```python
from build123d import *

# Parameters (mm, degrees)
BOSS_EXTRUDE1_DEPTH = 35.687
FILLET1_R           = 6.35
SKETCH3_R           = 4.1656
CUT_EXTRUDE1_DEPTH  = 114.518465322
CUT_EXTRUDE2_REACH  = 115.518
SKETCH4_R           = 4.1656


with BuildPart() as part:
    # Sketch2 → Boss-Extrude1 (new, symmetric)
    with BuildSketch(Plane.XY):
        with BuildLine():
            Line((0, 0), (0, 76.2))
            Line((0, 76.2), (6.35, 76.2))
            Line((6.35, 76.2), (6.35, 14.2748))
            ThreePointArc((6.35, 14.2748), (8.67112018, 8.67112018), (14.2748, 6.35))
            Line((14.2748, 6.35), (76.2, 6.35))
            Line((76.2, 6.35), (76.2, 0))
            Line((76.2, 0), (0, 0))
        make_face()
    extrude(amount=BOSS_EXTRUDE1_DEPTH, both=True)

    # Fillet1
    fillet1_edges = [part.edges().sort_by_distance(p)[0] for p in [
        (76.2, 6.35, 0),
        (6.35, 76.2, 0),
    ]]
    fillet(fillet1_edges, radius=FILLET1_R - 0.0001)  # a hair under: the kernel refuses the full size

    # Sketch3 → Cut-Extrude1 (cut, through all)
    with BuildSketch(Plane.ZY):
        with Locations(Location((-19.05, 57.15, 0), (0, 0, 270))):
            Circle(SKETCH3_R)
        with Locations(Location((-19.05, 19.05, 0), (0, 0, 270))):
            Circle(SKETCH3_R)
        with Locations(Location((19.05, 19.05, 0), (0, 0, 270))):
            Circle(SKETCH3_R)
        with Locations(Location((19.05, 57.15, 0), (0, 0, 270))):
            Circle(SKETCH3_R)
    extrude(amount=-CUT_EXTRUDE1_DEPTH, mode=Mode.SUBTRACT)

    # Sketch4 → Cut-Extrude2 (cut, up to next)
    with BuildSketch(Plane.XZ, mode=Mode.PRIVATE) as cut_extrude2_sk1:
        with Locations((57.15, 19.05)):
            Circle(SKETCH4_R)
    cut_extrude2_tool1 = extrude(cut_extrude2_sk1.sketch, amount=-CUT_EXTRUDE2_REACH, mode=Mode.PRIVATE) & part.part
    # Sketch4 → Cut-Extrude2 (cut, up to next)
    with BuildSketch(Plane.XZ, mode=Mode.PRIVATE) as cut_extrude2_sk2:
        with Locations(Location((19.05, -19.05, 0), (0, 0, 270))):
            Circle(SKETCH4_R)
    cut_extrude2_tool2 = extrude(cut_extrude2_sk2.sketch, amount=-CUT_EXTRUDE2_REACH, mode=Mode.PRIVATE) & part.part
    # Sketch4 → Cut-Extrude2 (cut, up to next)
    with BuildSketch(Plane.XZ, mode=Mode.PRIVATE) as cut_extrude2_sk3:
        with Locations(Location((57.15, -19.05, 0), (0, 0, 270))):
            Circle(SKETCH4_R)
    cut_extrude2_tool3 = extrude(cut_extrude2_sk3.sketch, amount=-CUT_EXTRUDE2_REACH, mode=Mode.PRIVATE) & part.part
    # Sketch4 → Cut-Extrude2 (cut, up to next)
    with BuildSketch(Plane.XZ, mode=Mode.PRIVATE) as cut_extrude2_sk4:
        with Locations((19.05, 19.05)):
            Circle(SKETCH4_R)
    cut_extrude2_tool4 = extrude(cut_extrude2_sk4.sketch, amount=-CUT_EXTRUDE2_REACH, mode=Mode.PRIVATE) & part.part
    add(cut_extrude2_tool1.solids().sort_by_distance((57.15, 0, 19.05))[0], mode=Mode.SUBTRACT)
    add(cut_extrude2_tool2.solids().sort_by_distance((19.05, 0, -19.05))[0], mode=Mode.SUBTRACT)
    add(cut_extrude2_tool3.solids().sort_by_distance((57.15, 0, -19.05))[0], mode=Mode.SUBTRACT)
    add(cut_extrude2_tool4.solids().sort_by_distance((19.05, 0, 19.05))[0], mode=Mode.SUBTRACT)


solid = part.part
```
Geometry: final body of the model. Coordinates: model frame, mm. A direction names the side the tool comes from. Coordinates: 2 decimals unless noted, no trailing zeros. Order: outer loops, then holes, each group sorted by start corner. A loop starts at its lowest first (then second) coordinate and runs counter-clockwise, first axis right, second up. Notation, with made-up numbers: M 2.25,64.25 L 61.25,64.25 A30 ccw 61.25,102.25 Z; hole C 37.25,26 d4. An arc over 180 degrees is marked long. Answer in a Markdown table with one row per item. Add a question column.
Q1. Contact query for flat-ended pins moving along their axis: P1, Ø9.5, axis at y = 19.05, z = 19.05, coming from the +X side; P2, Ø5, axis at x = 19.05, z = 19.05, coming from the +Y side; P3, Ø8, axis at x = 38.5, z = -9, coming from the -Y side. Output: stop coordinate, or through.
Q2. Line query: L1, parallel to Z at x = 57, y = 3; L2, parallel to Y at x = 2, z = -19; L3, parallel to Y at x = 32, z = 16. Output: solid intervals per line, ascending.
Q3. Mould query, pull axis X, two halves, no side actions, for faces 3 (the cylindrical face through (60.66, 3.13, -21.29)), 4 (the cylindrical face through (74.39, 4.44, 0.5)), 5 (the cylindrical face through (3.131, 58.053, 14.983)). Classes: released by +X, released by -X, zero draft, split by the parting line, or undercut.
Q4. Section query A-A on x = 57.15. Return the cut outline in (y, z), and give its area (3 significant figures).
Q5. Section query B-B on z = -19.05. Count the separate pieces of the cut face and the enclosed holes in it, and give its area (3 significant figures).
Q6. Reachability of faces 1 (the flat face through (6.35, 42, 0)), 2 (the cylindrical face through (53.84, 3.13, 16.52)) from +Z, -Z, +X, -X, +Y, -Y: full face, straight path, thin tool, end or side. Return the list, or none.
Completed:
| question | item | result |
|---|---|---|
| 1 | P1 | stops at x = 6.35 |
| 1 | P2 | passes through |
| 1 | P3 | stops at y = 0 |
| 2 | L1 | z = -35.69 to -23.21, -14.89 to 14.89, 23.21 to 35.69 |
| 2 | L2 | y = 0 to 14.88, 23.22 to 52.98, 61.32 to 75.88 |
| 2 | L3 | y = 0 to 6.35 |
| 3 | face 3 | undercut |
| 3 | face 4 | released by +X |
| 3 | face 5 | zero draft |
| 4 | outline | M 0,-35.69 L 6.35,-35.69 L 6.35,-23.22 L 0,-23.22 Z; M 0,-14.88 L 6.35,-14.88 L 6.35,14.88 L 0,14.88 Z; M 0,23.22 L 6.35,23.22 L 6.35,35.69 L 0,35.69 Z |
| 4 | area | 347 mm2 |
| 5 | separate pieces | 5 |
| 5 | enclosed holes | 0 |
| 5 | area | 712 mm2 |
| 6 | face 1 | +Z, -Z, +X, +Y |
| 6 | face 2 | +Y, -Y |
